Could you check a few things on this drawing? It's one solid part, dimensions in mm from its lowest x, y, z. A direction names the side the tool comes from. Give positions to 0.01 mm unless a question says otherwise; leave off trailing zeros. Loops run counter-clockwise (first coordinate to the right, second up) from the corner with the lowest first, then second, coordinate; pieces in that order, holes last. Notation, with made-up numbers: (21.5, -35) - (68.5, -35) arc R20 ccw to (68.5, -23) - close; hole circle Ø11 at (77.5, -15.5). An arc over 180 degrees is marked (long way). Write each question's results on one line, items separated by ' | '. Start each with the question number.
(1) On a 3-axis mill with a long thin cutter (end or side, diameter ignored), from which of +Z, -Z, +X, -X, +Y, -Y can I reach the whole of each face in a straight line? I mean the marked faces 4, 5, 6 and 7. Say none if no direction works.
(2) For pin 1 (6 mm diameter, centred on x = 21, z = 6.5, fed in from -Y); pin 2 (1 mm diameter, centred on x = 5, z = 9.5, fed in from -Y); pin 3 (1.2 mm diameter, centred on x = 36, y = 12, fed in from +Z); pin 4 (0.8 mm diameter, centred on x = 36, y = 11.5, fed in from -Z), each with a flat end and sliding along its axis, tell me the tip position at first contact or that it passes through.
(3) Suppose I cut it at D-D (y = 14.25). Please give me the cut outline in (x, z), and give its area (3 significant figures).
(4) Suppose I cut it at C-C (z = 12). Please give me the cut outline in (x, y).
(5) Suppose I cut it at B-B (z = 19.25). Please give me the cut outline in (x, y).
(6) If we mould it in two halves opening along X, with no side actions, what happens to the marked faces 1, 2 and 3? For each: released by +X, released by -X, zero draft, split by the parting line, or undercut.
(7) Suppose I cut it at A-A (x = 2.5). Please give me the cut outline in (y, z).
(8) I need wall thicknesses on line 1 (Z direction, x = 2.5, y = 6.2); line 2 (X direction, y = 6.75, z = 19.5); line 3 (Y direction, x = 30.5, z = 1.75). Which ranges of each line are inside material? Lowest first, please.
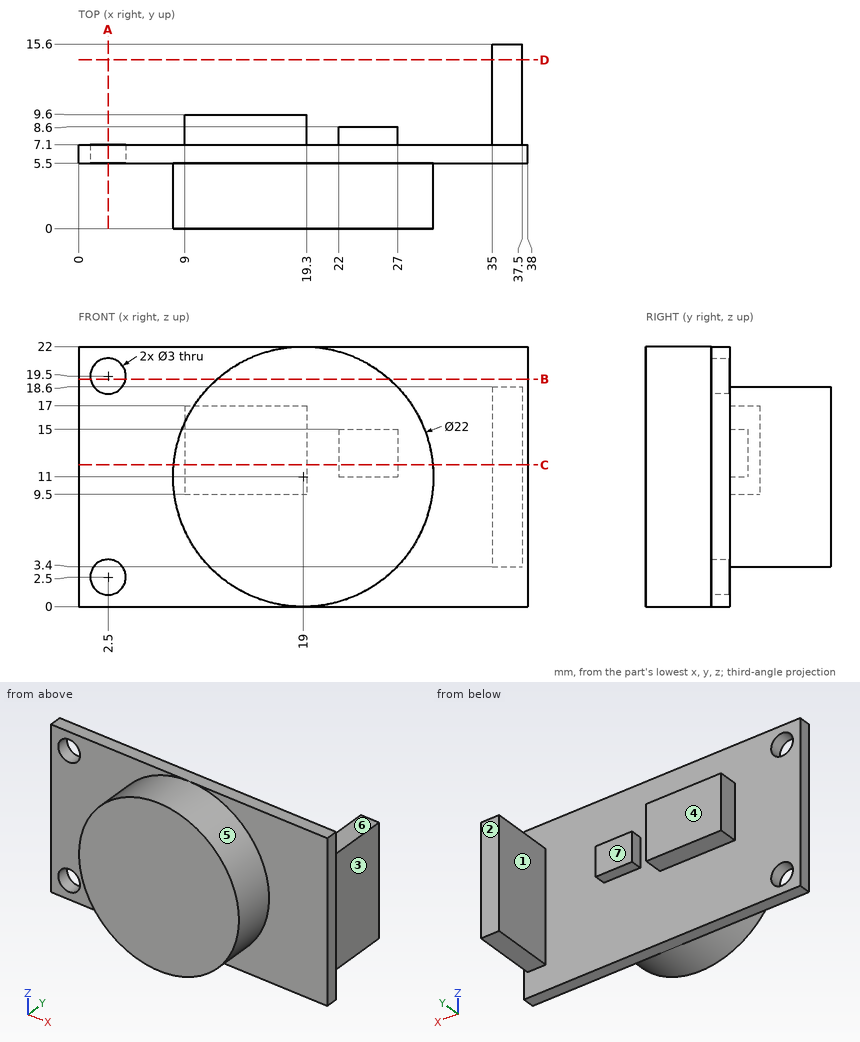
Output values:
1) face 4: +Z, -Z, -X, +Y | face 5: -Y | face 6: +Z, +X, -X, +Y | face 7: +Z, -Z, +Y
2) pin 1: y = 0 | pin 2: y = 5.5 | pin 3: z = 18.6 | pin 4: z = 3.4
3) outline: (35, 3.4) - (37.5, 3.4) - (37.5, 18.6) - (35, 18.6) - close | area: 38.0 mm2
4) outline: (0, 5.5) - (8.05, 5.5) - (8.05, 0) - (29.95, 0) - (29.95, 5.5) - (38, 5.5) - (38, 7.1) - (37.5, 7.1) - (37.5, 15.6) - (35, 15.6) - (35, 7.1) - (27, 7.1) - (27, 8.6) - (22, 8.6) - (22, 7.1) - (19.3, 7.1) - (19.3, 9.6) - (9, 9.6) - (9, 7.1) - (0, 7.1) - close
5) outline: (0, 5.5) - (1.02, 5.5) - (1.02, 7.1) - (0, 7.1) - close; (3.98, 5.5) - (11.72, 5.5) - (11.72, 0) - (26.28, 0) - (26.28, 5.5) - (38, 5.5) - (38, 7.1) - (3.98, 7.1) - close
6) face 1: undercut | face 2: zero draft | face 3: released by +X
7) outline: (5.5, 0) - (7.1, 0) - (7.1, 1) - (5.5, 1) - close; (5.5, 4) - (7.1, 4) - (7.1, 18) - (5.5, 18) - close; (5.5, 21) - (7.1, 21) - (7.1, 22) - (5.5, 22) - close
8) line 1: 0 to 1, 4 to 18, 21 to 22 | line 2: 0 to 1, 4 to 38 | line 3: 5.5 to 7.1
